```python
from build123d import *

# Parameters (mm, degrees)
SKETCH1_W           = 44.45
SKETCH1_H           = 3.175
BOSS_EXTRUDE1_DEPTH = 6.35
SKETCH2_R           = 2.4003
CUT_EXTRUDE1_DEPTH  = 8.89
FILLET1_R           = 0.635
SKETCH4_R           = 0.889
CUT_EXTRUDE2_DEPTH  = 3.81


with BuildPart() as part:
    # Sketch1 → Boss-Extrude1 (new body)
    with BuildSketch(Plane(origin=(0, 0, 0), x_dir=(1, 0, 0), z_dir=(0, 1, 0))):
        with Locations((22.225, 4.7625)):
            Rectangle(SKETCH1_W, SKETCH1_H)
        with Locations((22.225, 1.5875)):
            Rectangle(SKETCH1_W, SKETCH1_H)
        Polygon((44.45, 6.35), (44.45, 3.175), (57.15, 3.175), (44.45, 9.525), align=None)
        Polygon((57.15, 3.175), (44.45, 3.175), (44.45, 0), (44.45, -3.175), align=None)
    extrude(amount=BOSS_EXTRUDE1_DEPTH)

    # Sketch2 → Cut-Extrude1 (cut)
    with BuildSketch(Plane.ZY):
        with Locations((-3.175, 3.175)):
            Circle(SKETCH2_R)
    extrude(amount=-CUT_EXTRUDE1_DEPTH, mode=Mode.SUBTRACT)

    # Fillet1
    fillet1_edges = [part.edges().sort_by_distance(p)[0] for p in [
        (0, 3.175, -6.35),
        (44.45, 3.175, -6.35),
        (44.45, 3.175, -9.525),
        (57.15, 3.175, -3.175),
        (44.45, 3.175, 3.175),
        (44.45, 3.175, 0),
        (0, 3.175, 0),
    ]]
    fillet(fillet1_edges, radius=FILLET1_R)

    # Sketch4 → Cut-Extrude2 (cut)
    with BuildSketch(Plane.XZ):
        with Locations(Location((20.562548417, -3.175, 0), (0, 0, 270))):
            Circle(SKETCH4_R)
        with Locations(Location((35.802548417, -3.175, 0), (0, 0, 270))):
            Circle(SKETCH4_R)
    extrude(amount=-CUT_EXTRUDE2_DEPTH, mode=Mode.SUBTRACT)


solid = part.part
```
Geometry: final body of the model. Coordinates: model frame, mm. A direction names the side the tool comes from. Round coordinates to 2 decimals unless told otherwise and drop trailing zeros. Loops run counter-clockwise (first coordinate to the right, second up) from the corner with the lowest first, then second, coordinate; pieces in that order, holes last. Notation, with made-up numbers: (34.5, 13) -> (86.5, 13) arc R21 ccw to (86.5, 34) -> close; hole circle Ø6 at (12.5, 47). An arc over 180 degrees is marked (long way). Use one line per item in the form item = value.
Item 1: Cut plane A-A on y = 2. Give the number of separate pieces and of enclosed holes in the cut face, then the cut area to 3 significant figures.
Evaluation:
separate_pieces = 1
enclosed_holes = 2
area = 320 mm2
Item 2: Contact query for flat-ended pins moving along their axis: pin 1 Ø1.2 at (y, z) = (3, 2) entering from -X; pin 2 Ø1.4 at (y, z) = (4, -4) entering from -X; pin 3 Ø0.9 at (x, z) = (36, -3) entering from -Y. Output: stop coordinate, or through.
Evaluation:
pin_1 = 44.45
pin_2 = 8.89
pin_3 = 3.81
Item 3: Cut plane D-D on x = 50. Output: boundary loops of the cut face in (y, z), then the cut area to 3 significant figures.
Evaluation:
outline = (0, -6.75) -> (6.35, -6.75) -> (6.35, 0.4) -> (0, 0.4) -> close
area = 45.4 mm2
Item 4: Cut plane C-C on z = -8. Output: boundary loops of the cut face in (x, y).
Evaluation:
outline = (44.45, 0) -> (47.5, 0) -> (47.5, 6.35) -> (44.45, 6.35) -> close
Item 5: Cut plane B-B on x = 6. Output: boundary loops of the cut face in (y, z) (3 decimals).
Evaluation:
outline = (0, -6.35) -> (6.35, -6.35) -> (6.35, 0) -> (0, 0) -> close; hole circle Ø4.801 at (3.175, -3.175)
Item 6: Access query for faces 1 (the flat face through (21, 3.81, -3)), 2 (the cylindrical face through (4.383, 3.896, -0.886)), 3 (the flat face through (44.45, 3, 1)), 4 (the flat face through (44.45, 3, -8)), 5 (the cylindrical face through (44.74, 3.22, -9.03)). Directions: +Z, -Z, +X, -X, +Y, -Y. A direction counts if a zero-diameter tool reaches every point of the face in a straight line with its end or side. Return the directions, or none.
Evaluation:
face_1 = -Y
face_2 = -X
face_3 = +Z, -X, +Y, -Y
face_4 = -Z, -X, +Y, -Y
face_5 = -Z, +Y, -Y
Item 7: Draft query along X for faces 6 (the cylindrical face through (56.365, 3.219, -3.165)), 7 (the flat face through (36, 3.81, -3)), 8 (the flat face through (22, 3, -6.35)). Return one class per face: released by +X, released by -X, zero draft, split by the parting line, or undercut.
Evaluation:
face_6 = released by +X
face_7 = undercut
face_8 = zero draft
Item 8: Material intervals for probe 1 along Z at (x, y) = (12, 0.5); probe 2 along Z at (x, y) = (4, 1); probe 3 along Z at (x, y) = (4, 3.5), sorted ascending.
Evaluation:
probe_1 = -6.35 to 0
probe_2 = -6.35 to -4.19, -2.16 to 0
probe_3 = -6.35 to -5.55, -0.8 to 0
